```python
from build123d import *

# Parameters (mm, degrees)
SKETCH1_W               = 155
SKETCH1_H               = 55
EXTRUDE1_DEPTH          = 3
FILLET1_R               = 25
TAB_AND_SLOT_TAB1_DEPTH = 3


# Read off the part's stored shape, not the designer's step: Tab and Slot-Tab1
with BuildPart() as part:
    # Sketch1 → Extrude1 (new body)
    with BuildSketch(Plane(origin=(0, 0, 0), x_dir=(1, 0, 0), z_dir=(0, 1, 0))):
        Rectangle(SKETCH1_W, SKETCH1_H)
        with BuildLine():
            Line((-50, 17.5), (50, 17.5))
            ThreePointArc((50, 17.5), (62.5, 5), (50, -7.5))
            Line((50, -7.5), (-50, -7.5))
            ThreePointArc((-50, -7.5), (-62.5, 5), (-50, 17.5))
        make_face(mode=Mode.SUBTRACT)
    extrude(amount=EXTRUDE1_DEPTH)

    # Fillet1
    fillet1_edges = [part.edges().sort_by_distance(p)[0] for p in [
        (-77.5, 1.5, -27.5),
        (77.5, 1.5, -27.5),
    ]]
    fillet(fillet1_edges, radius=FILLET1_R)

    # Tab and Slot-Tab1 outline → Tab and Slot-Tab1 (add)
    with BuildSketch(Plane(origin=(0, 0, 0), x_dir=(1, 0, 0), z_dir=(0, 1, 0))):
        Polygon((62.5, -27.5), (42.5, -27.5), (42.5, -29.5), (43.5, -30.5), (61.5, -30.5), (62.5, -29.5), align=None)
        Polygon((-42.5, -29.5), (-42.5, -27.5), (-62.5, -27.5), (-62.5, -29.5), (-61.5, -30.5), (-43.5, -30.5), align=None)
    extrude(amount=TAB_AND_SLOT_TAB1_DEPTH)


solid = part.part
```
Source: CAD feature listing. Evaluate the final solid. Frame: model axes, mm. A direction names the side the tool comes from. Give positions to 0.01 mm unless a question says otherwise; leave off trailing zeros. Loops run counter-clockwise (first coordinate to the right, second up) from the corner with the lowest first, then second, coordinate; pieces in that order, holes last. Notation, with made-up numbers: (-39, 86.25) -> (20, 86.25) arc R17 ccw to (20, 114.25) -> close; hole circle Ø10 at (53.25, 68.5). An arc over 180 degrees is marked (long way). Put each result on its own line as item: value. Start each with the question number.
1) Cut plane C-C (z = -4.5). Return loops of the section in (x, y).
2) Cut plane B-B (y = 2.1). Return loops of the section in (x, z).
3) Cut plane D-D (z = -19). Return loops of the section in (x, y), then the cut area to 3 significant figures.
4) Draft query along X for faces 1 (the face through (-70.371, 1.521, -19.982)), 2 (the face through (-1, 1, 27.5)), 3 (the face through (52, 1, 30.5)), 4 (the face through (69.982, 1.521, -20.371)). Return one class per face: released by +X, released by -X, zero draft, split by the parting line, or undercut.
5) Reachability of faces 5 (the face through (-70, 1, 27.5)), 6 (the face through (77.5, 1, 13)), 7 (the face through (70, 1, 27.5)), 8 (the face through (62.497, 1.479, -5.275)) from +Z, -Z, +X, -X, +Y, -Y: full face, straight path, thin tool, end or side. Return the list, or none.
6) Material intervals for probe 1 along Z at (x, y) = (6, 0.5); probe 2 along Z at (x, y) = (-49, 1.85); probe 3 along X at (y, z) = (1.75, -11.5), sorted ascending.
7) Contact query for flat-ended pins moving along their axis: P1, Ø1, axis at x = -22.5, z = 8.5, coming from the -Y side; P2, Ø0.6, axis at y = 1.5, z = 29, coming from the -X side; P3, Ø0.6, axis at y = 2, z = 28.5, coming from the +X side; P4, Ø2, axis at x = -39.5, z = 5.5, coming from the -Y side. Output: stop coordinate, or through.
8) Cut plane A-A (x = 12). Return loops of the section in (y, z).
Results are:
1. outline: (-77.42, 0) -> (-62.49, 0) -> (-62.49, 3) -> (-77.42, 3) -> close; (62.49, 0) -> (77.42, 0) -> (77.42, 3) -> (62.49, 3) -> close
2. outline: (-77.5, -2.5) arc R25 ccw to (-52.5, -27.5) -> (52.5, -27.5) arc R25 ccw to (77.5, -2.5) -> (77.5, 27.5) -> (62.5, 27.5) -> (62.5, 29.5) -> (61.5, 30.5) -> (43.5, 30.5) -> (42.5, 29.5) -> (42.5, 27.5) -> (-42.5, 27.5) -> (-42.5, 29.5) -> (-43.5, 30.5) -> (-61.5, 30.5) -> (-62.5, 29.5) -> (-62.5, 27.5) -> (-77.5, 27.5) -> close; hole (-50, -17.5) -> (50, -17.5) arc R12.5 ccw to (50, 7.5) -> (-50, 7.5) arc R12.5 ccw to start
3. outline: (-71.28, 0) -> (71.28, 0) -> (71.28, 3) -> (-71.28, 3) -> close
3. area: 428 mm2
4. face 1: released by -X
4. face 2: undercut
4. face 3: zero draft
4. face 4: released by +X
5. face 5: +Z, -X, +Y, -Y
5. face 6: +Z, -Z, +X, +Y, -Y
5. face 7: +Z, +X, +Y, -Y
5. face 8: +Y, -Y
6. probe 1: z = -27.5 to -17.5, 7.5 to 27.5
6. probe 2: z = -27.5 to -17.5, 7.5 to 30.5
6. probe 3: x = -75.82 to -60.68, 60.68 to 75.82
7. P1: stops at y = 0
7. P2: stops at x = -62.5
7. P3: stops at x = 62.5
7. P4: passes through
8. outline: (0, -27.5) -> (3, -27.5) -> (3, -17.5) -> (0, -17.5) -> close; (0, 7.5) -> (3, 7.5) -> (3, 27.5) -> (0, 27.5) -> close
